The listing builds one solid part. Answer for the finished solid, in the listing's coordinates (mm). A direction names the side the tool comes from. Give positions to 0.01 mm unless a question says otherwise; leave off trailing zeros. Order: outer loops, then holes, each group sorted by start corner. A loop starts at its lowest first (then second) coordinate and runs counter-clockwise, first axis right, second up. Notation, with made-up numbers: M 62,-36 L 98,-36 A29 ccw 98,-14 Z; hole C 40,82 d6. An arc over 180 degrees is marked long. Answer as a JSON object with one key per item and string values. Group by question number.
```python
from build123d import *

# Parameters (mm, degrees)
BOSS_EXTRUDE3_DEPTH      = 25
BOSS_EXTRUDE3_DEPTH_BACK = 14.3
SKETCH6_R                = 26.15
BOSS_EXTRUDE4_DEPTH      = 90
SKETCH7_R                = 10.75
SKETCH7_R_2              = 8.15
BOSS_EXTRUDE5_DEPTH      = 5
SKETCH8_R                = 9
BOSS_EXTRUDE6_DEPTH      = 7
SKETCH9_R                = 22.25
SKETCH9_R_2              = 17.5
SKETCH9_R_3              = 26.15
BOSS_EXTRUDE7_DEPTH      = 35
SKETCH10_R               = 17.5
SKETCH10_R_2             = 15
BOSS_EXTRUDE8_DEPTH      = 425
FILLET1_R                = 2


with BuildPart() as part:
    # Sketch5 → Boss-Extrude3 (new body, two sides)
    with BuildSketch(Plane(origin=(0, 0, 0), x_dir=(1, 0, 0), z_dir=(0, 1, 0))) as boss_extrude3_sk:
        with BuildLine():
            Line((-52, -32), (42, -32))
            add(Edge.make_bspline(
                [(42, 42), (69.3, 5), (42, -32)],
                knots=[0, 0, 0, 1, 1, 1], degree=2))
            Line((42, 42), (-52, 42))
            add(Edge.make_bspline(
                [(-52, 42), (-79.3, 5), (-52, -32)],
                knots=[0, 0, 0, 1, 1, 1], degree=2))
        make_face()
    extrude(amount=BOSS_EXTRUDE3_DEPTH)
    extrude(boss_extrude3_sk.sketch, amount=-BOSS_EXTRUDE3_DEPTH_BACK)

    # Sketch6 → Boss-Extrude4 (add)
    with BuildSketch(Plane(origin=(0, 25, 0), x_dir=(1, 0, 0), z_dir=(0, 1, 0))):
        with Locations((29.05, 5)):
            Circle(SKETCH6_R)
    extrude(amount=BOSS_EXTRUDE4_DEPTH)

    # Sketch7 → Boss-Extrude5 (add)
    with BuildSketch(Plane(origin=(0, 115, 0), x_dir=(1, 0, 0), z_dir=(0, 1, 0))):
        with Locations((29.05, 5)):
            Circle(SKETCH7_R)
        with Locations((29.05, 5)):
            Circle(SKETCH7_R_2, mode=Mode.SUBTRACT)
    extrude(amount=BOSS_EXTRUDE5_DEPTH)

    # Sketch8 → Boss-Extrude6 (add)
    with BuildSketch(Plane(origin=(0, 115, 0), x_dir=(1, 0, 0), z_dir=(0, 1, 0))):
        with Locations((29.05, 5)):
            Circle(SKETCH8_R)
    extrude(amount=BOSS_EXTRUDE6_DEPTH)

    # Sketch9 → Boss-Extrude7 (add)
    with BuildSketch(Plane(origin=(0, 25, 0), x_dir=(1, 0, 0), z_dir=(0, 1, 0))):
        with Locations((-29.55, 5)):
            Circle(SKETCH9_R)
        with Locations((-29.55, 5)):
            Circle(SKETCH9_R_2, mode=Mode.SUBTRACT)
        with Locations((29.05, 5)):
            Circle(SKETCH9_R_3)
    extrude(amount=BOSS_EXTRUDE7_DEPTH)

    # Sketch10 → Boss-Extrude8 (add)
    with BuildSketch(Plane(origin=(0, 25, 0), x_dir=(1, 0, 0), z_dir=(0, 1, 0))):
        with Locations((-29.55, 5)):
            Circle(SKETCH10_R)
        with Locations((-29.55, 5)):
            Circle(SKETCH10_R_2, mode=Mode.SUBTRACT)
    extrude(amount=BOSS_EXTRUDE8_DEPTH)

    # Fillet1
    fillet1_edges = [part.edges().sort_by_distance(p)[0] for p in [
        (42, 12.5, -42),
        (-52, 12.5, -42),
        (-52, 12.5, 32),
        (42, 12.5, 32),
    ]]
    fillet(fillet1_edges, radius=FILLET1_R)


solid = part.part
```
Item 1: Section C-C (x = 29.05) is taken. Determine the outline of the cut face in (y, z).
Item 2: Flat-ended cylindrical pins translate along their axes: P1, Ø1.5, axis at y = 364.5, z = -10.5, coming from the -X side; P2, Ø8, axis at x = -47, y = 230, coming from the +Z side; P3, Ø4, axis at y = 362, z = -21.5, coming from the +X side. Find the tip coordinate at first contact, or state that the pin passes through.
Item 3: Consider probe 1 along X at (y, z) = (45.5, -6.5); probe 2 along X at (y, z) = (295, -5); probe 3 along Z at (x, y) = (-29, 252). Determine where each line is inside the solid, lowest interval first. Write a range as from..to.
Item 4: Section B-B (x = -29.55) is taken. Determine the outline of the cut face in (y, z), and give its area (3 significant figures).
Item 5: Section A-A (y = 31.5) is taken. Determine the outline of the cut face in (x, z).
Item 6: Section D-D (y = 221) is taken. Determine the outline of the cut face in (x, z).
Item 7: Determine the mould class of faces 4 (the flat face through (40, 115, -5)), 5 (the flat face through (-6, 6, 32)) for opening direction X: released by +X, released by -X, zero draft, split by the parting line, or undercut.
Item 8: A tool of negligible diameter and unlimited length cuts with its end or side. For faces 1 (the flat face through (29, 122, -5)), 2 (the flat face through (-15, 450, -10)), 3 (the cylindrical face through (-47.207, 42.255, 8.539)), from which of +Z, -Z, +X, -X, +Y, -Y can it reach the whole face along a straight path? Write none if from no direction.
Values found:
{
 "1": {"outline": "M -14.3,-42 L 25,-42 L 25,-31.15 L 115,-31.15 L 115,-15.75 L 120,-15.75 L 120,-14 L 122,-14 L 122,4 L 120,4 L 120,5.75 L 115,5.75 L 115,21.15 L 25,21.15 L 25,32 L -14.3,32 Z"},
 "2": {"P1": "stops at x = -46.39", "P2": "stops at z = 6.2", "P3": "stops at x = -19.75"},
 "3": {"probe 1": "x = -51.75..-44.47, -14.63..-7.35, 2.94..55.16", "probe 2": "x = -47.05..-44.55, -14.55..-12.05", "probe 3": "z = -22.49..-19.99, 9.99..12.49"},
 "4": {"outline": "M -14.3,-42 L 25,-42 L 25,-27.25 L 60,-27.25 L 60,-22.5 L 450,-22.5 L 450,-20 L 25,-20 L 25,10 L 450,10 L 450,12.5 L 60,12.5 L 60,17.25 L 25,17.25 L 25,32 L -14.3,32 Z", "area": "5,370 mm^2"},
 "5": {"outline": "C -29.55,-5 d44.5; C 29.05,-5 d52.3; hole C -29.55,-5 d30"},
 "6": {"outline": "C -29.55,-5 d35; hole C -29.55,-5 d30"},
 "7": {"face 4": "undercut", "face 5": "zero draft"},
 "8": {"face 1": "+Z, -Z, +X, +Y", "face 2": "+Z, -Z, +X, -X, +Y", "face 3": "+Y"}
}
